Input: part model. Units: mm. Frame: model coordinates. A direction names the side the tool comes from. Give positions to 0.01 mm unless a question says otherwise; leave off trailing zeros. Loops run counter-clockwise (first coordinate to the right, second up) from the corner with the lowest first, then second, coordinate; pieces in that order, holes last. Notation, with made-up numbers: (-2, 85) -> (15, 85) arc R7 cw to (15, 93) -> close; hole circle Ø3 at (66, 16.5). An arc over 180 degrees is marked (long way). Answer in a Markdown table with one row per item. Add a question column.
```python
from build123d import *

# Parameters (mm, degrees)
SKETCH1_R         = 10.55
SKETCH1_R_2       = 9
EXTRUDE1_DEPTH    = 5
EXTRUDE1_DRAFT    = 1.5
EXTRUDE3_DEPTH    = 1.5
CIRPATTERN1_COUNT = 4
SKETCH5_R         = 0.75
EXTRUDE4_DEPTH    = 1
SKETCH6_R         = 1.5
EXTRUDE5_DEPTH    = 1


with BuildPart() as part:
    # Sketch1 → Extrude1 (with draft: the straight prism first)
    with BuildSketch(Plane(origin=(0, 0, 0), x_dir=(1, 0, 0), z_dir=(0, 1, 0))):
        Circle(SKETCH1_R)
        Circle(SKETCH1_R_2, mode=Mode.SUBTRACT)
    extrude(amount=EXTRUDE1_DEPTH)
    # Extrude1: the draft: its side faces are tilted about the plane it starts from
    extrude1_sides = [part.faces().sort_by_distance(p)[0] for p in [
        (-10.55, 2.5, 0),
        (-9, 2.5, 0),
    ]]
    draft(extrude1_sides, Plane(origin=(0, 0, 0), x_dir=(1, 0, 0), z_dir=(0, 1, 0)), EXTRUDE1_DRAFT)

    # Sketch4 → Extrude3 (add)
    with BuildSketch(Plane(origin=(0, 5, 0), x_dir=(1, 0, 0), z_dir=(0, 1, 0))):
        with BuildLine():
            Line((-1, 9.5), (1, 9.5))
            Line((1, 9.5), (1, 1.732050808))
            ThreePointArc((1, 1.732050808), (0, -2), (-1, 1.732050808))
            Line((-1, 1.732050808), (-1, 9.5))
        make_face()
    extrude3 = extrude(amount=-EXTRUDE3_DEPTH)

    # CirPattern1: Extrude3 ×4 about axis
    cirpattern1_axis = Axis((0, 0, 0), (0, 1, 0))
    for i in range(1, CIRPATTERN1_COUNT):
        add(extrude3.rotate(cirpattern1_axis, i * 360 / CIRPATTERN1_COUNT))

    # Sketch5 → Extrude4 (add)
    with BuildSketch(Plane(origin=(0, 5, 0), x_dir=(1, 0, 0), z_dir=(0, 1, 0))):
        with Locations(Location((0, 0, 0), (0, 0, 270))):
            Circle(SKETCH5_R)
    extrude(amount=EXTRUDE4_DEPTH)

    # Sketch6 → Extrude5 (add)
    with BuildSketch(Plane(origin=(0, 6, 0), x_dir=(1, 0, 0), z_dir=(0, 1, 0))):
        with Locations(Location((0, 0, 0), (0, 0, 270))):
            Circle(SKETCH6_R)
    extrude(amount=EXTRUDE5_DEPTH)


solid = part.part
```
1) Section A-A on x = 0. Output: boundary loops of the cut face in (y, z).
2) Pin query (flat end, axial travel): pin 1 (2 mm diameter, centred on x = -8, z = 7.5, fed in from +Y); pin 2 (1.6 mm diameter, centred on x = 6.5, y = 4, fed in from +Z); pin 3 (0.8 mm diameter, centred on x = 5.5, y = 4.5, fed in from -Z); pin 4 (1 mm diameter, centred on y = 6, z = -4, fed in from -X). Return the tip coordinate at first contact, or that it passes through.
3) Reachability of faces 1 (the face through (8, 0, -5)), 2 (the face through (0.45, 6.49, 1.43)) from +Z, -Z, +X, -X, +Y, -Y: full face, straight path, thin tool, end or side. Return the list, or none.
4) Section D-D on x = -8.5. State how many separate pieces and enclosed holes the cut face has, and give its area (3 significant figures).
5) Section B-B on z = 0. Output: boundary loops of the cut face in (x, y).
6) Section C-C on y = 4.5. Output: boundary loops of the cut face in (x, z).
7) Material intervals for line 1 along X through (y, z) = (4.5, -8); line 2 along X through (y, z) = (4.5, 4.75); line 3 along Y through (x, z) = (0.25, 0.75), sorted ascending.
8) Pull-direction query (Y, two-part tool) for faces 3 (the face through (5, 4, -1)), 4 (the face through (1, 6, 0)), 5 (the face through (10, 2.47, -3.15)), 6 (the face through (0.225, 5.493, 0.715)); classes: +Y half, -Y half, draft (parallel to the pull), parting line (faces both ways), or undercut.
Working result:
| question | item | result |
|---|---|---|
| 1 | outline | (0, -10.55) -> (5, -10.42) -> (5, -0.75) -> (6, -0.75) -> (6, -1.5) -> (7, -1.5) -> (7, 1.5) -> (6, 1.5) -> (6, 0.75) -> (5, 0.75) -> (5, 10.42) -> (0, 10.55) -> (0, 9) -> (3.5, 9.09) -> (3.5, -9.09) -> (0, -9) -> close |
| 2 | pin 1 | stops at y = 5 |
| 2 | pin 2 | stops at z = 8.75 |
| 2 | pin 3 | stops at z = -9.1 |
| 2 | pin 4 | passes through |
| 3 | face 1 | +Z, -Z, +X, -X, -Y |
| 3 | face 2 | +Y |
| 4 | separate pieces | 3 |
| 4 | enclosed holes | 0 |
| 4 | area | 32.9 mm2 |
| 5 | outline | (-10.55, 0) -> (-9, 0) -> (-9.09, 3.5) -> (9.09, 3.5) -> (9, 0) -> (10.55, 0) -> (10.42, 5) -> (0.75, 5) -> (0.75, 6) -> (1.5, 6) -> (1.5, 7) -> (-1.5, 7) -> (-1.5, 6) -> (-0.75, 6) -> (-0.75, 5) -> (-10.42, 5) -> close |
| 6 | outline | circle Ø20.86 at (0, 0); hole (-9.06, -1) arc R9.12 ccw to (-1, -9.06) -> (-1, -1.73) arc R2 cw to (-1.73, -1) -> close; hole (-9.06, 1) -> (-1.73, 1) arc R2 cw to (-1, 1.73) -> (-1, 9.06) arc R9.12 ccw to start; hole (1, -9.06) arc R9.12 ccw to (9.06, -1) -> (1.73, -1) arc R2 cw to (1, -1.73) -> close; hole (1, 1.73) arc R2 cw to (1.73, 1) -> (9.06, 1) arc R9.12 ccw to (1, 9.06) -> close |
| 7 | line 1 | x = -6.7 to -4.37, -1 to 1, 4.37 to 6.7 |
| 7 | line 2 | x = -9.29 to -7.78, -1 to 1, 7.78 to 9.29 |
| 7 | line 3 | y = 3.5 to 5, 6 to 7 |
| 8 | face 3 | draft |
| 8 | face 4 | undercut |
| 8 | face 5 | +Y half |
| 8 | face 6 | undercut |
